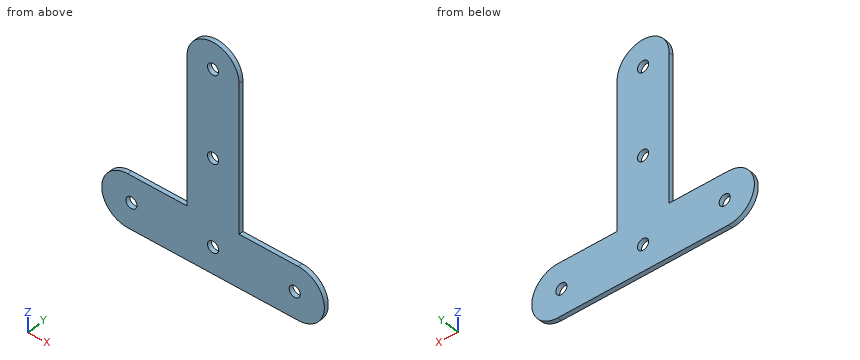
from build123d import *

# Parameters (mm, degrees)
SKETCH_1_R      = 1.5
EXTRUDE_1_DEPTH = 1.2


with BuildPart() as part:
    # 草图1 → 凸台-拉伸1 (new body)
    with BuildSketch(Plane(origin=(0, 0, 0), x_dir=(1, 0, 0), z_dir=(0, 1, 0))):
        with BuildLine():
            Line((-23, 7), (23, 7))
            ThreePointArc((23, 7), (30, 0), (23, -7))
            Line((23, -7), (7, -7))
            Line((7, -7), (7, -46))
            ThreePointArc((7, -46), (0, -53), (-7, -46))
            Line((-7, -46), (-7, -7))
            Line((-7, -7), (-23, -7))
            ThreePointArc((-23, -7), (-30, 0), (-23, 7))
        make_face()
        with Locations(Location((22, 0, 0), (0, 0, 270))):
            Circle(SKETCH_1_R, mode=Mode.SUBTRACT)
        with Locations(Location((-22, 0, 0), (0, 0, 270))):
            Circle(SKETCH_1_R, mode=Mode.SUBTRACT)
        with Locations(Location((0, 0, 0), (0, 0, 270))):
            Circle(SKETCH_1_R, mode=Mode.SUBTRACT)
        with Locations(Location((0, -23, 0), (0, 0, 270))):
            Circle(SKETCH_1_R, mode=Mode.SUBTRACT)
        with Locations(Location((0, -46, 0), (0, 0, 270))):
            Circle(SKETCH_1_R, mode=Mode.SUBTRACT)
    extrude(amount=EXTRUDE_1_DEPTH)


solid = part.part
Can you work these out from the model? Positions are in its coordinate system, mm. Coordinates: 2 decimals unless noted, no trailing zeros. Loops run counter-clockwise (first coordinate to the right, second up) from the corner with the lowest first, then second, coordinate; pieces in that order, holes last. Notation, with made-up numbers: M -18.5,-20.5 L 39.5,-20.5 A5 ccw 39.5,-13.5 Z; hole C -35.75,39.25 d8. An arc over 180 degrees is marked long. Answer as CSV lines item,"result". Start each with the question number.
1. If I drill on probe 1 along X at (y, z) = (0.3, 0); probe 2 along Z at (x, y) = (12.5, 0.45), over which ranges is the centre line in solid material (lowest first)? Write a range as [from, to].
2. Suppose I cut it at C-C, the plane z = 0. List the corners of the cut face in (x, y) for me.
3. Suppose I cut it at D-D, the plane x = 0. List the corners of the cut face in (y, z) for me.
4. For pin 1 Ø0.6 at (x, y) = (-17.5, 1) entering from +Z; pin 2 Ø2.5 at (x, z) = (0, 23) entering from +Y, each with a flat end and sliding along its axis, tell me the tip position at first contact or that it passes through.
5. Suppose I cut it at A-A, the plane x = 22. List the corners of the cut face in (y, z) for me.
6. Suppose I cut it at B-B, the plane y = 1. List the corners of the cut face in (x, z) for me, plus the area to 3 significant figures.
Output:
1,probe 1,"x = [-30, -23.5], [-20.5, -1.5], [1.5, 20.5], [23.5, 30]"
1,probe 2,"z = [-7, 7]"
2,outline,"M -30,0 L -23.5,0 L -23.5,1.2 L -30,1.2 Z; M -20.5,0 L -1.5,0 L -1.5,1.2 L -20.5,1.2 Z; M 1.5,0 L 20.5,0 L 20.5,1.2 L 1.5,1.2 Z; M 23.5,0 L 30,0 L 30,1.2 L 23.5,1.2 Z"
3,outline,"M 0,-7 L 1.2,-7 L 1.2,-1.5 L 0,-1.5 Z; M 0,1.5 L 1.2,1.5 L 1.2,21.5 L 0,21.5 Z; M 0,24.5 L 1.2,24.5 L 1.2,44.5 L 0,44.5 Z; M 0,47.5 L 1.2,47.5 L 1.2,53 L 0,53 Z"
4,pin 1,"stops at z = 7"
4,pin 2,"passes through"
5,outline,"M 0,-7 L 1.2,-7 L 1.2,-1.5 L 0,-1.5 Z; M 0,1.5 L 1.2,1.5 L 1.2,7 L 0,7 Z"
6,outline,"M -23,-7 L 23,-7 A7 ccw 23,7 L 7,7 L 7,46 A7 ccw -7,46 L -7,7 L -23,7 A7 ccw Z; hole C -22,0 d3; hole C 0,0 d3; hole C 0,23 d3; hole C 0,46 d3; hole C 22,0 d3"
6,area,"1,390 mm^2"
